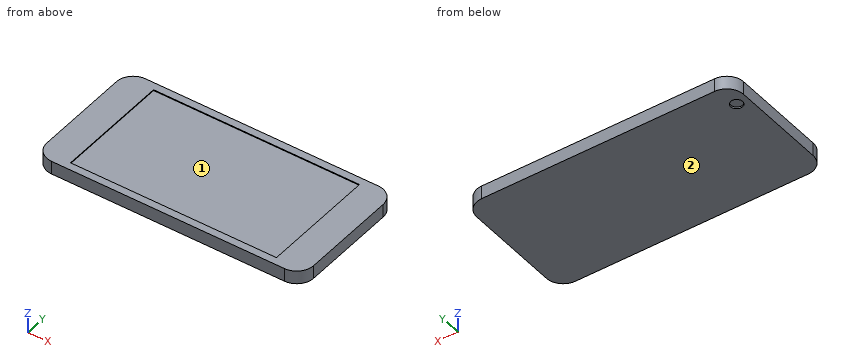
```python
from build123d import *

# Parameters (mm, degrees)
F0_W     = 158
F0_H     = 7.87
F1_DEPTH = 38.435
F2_R     = 10
F3_W     = 122
F3_H     = 68
F4_DEPTH = 0.5
F7_R     = 3.5
F8_DEPTH = 1


# Not quite as in the source:
# - the program builds the solid bodies; features that only make, move or delete a surface that nothing else refers to are left out


with BuildPart() as f1:
    # F0 (on Front) → F1 (new body, symmetric)
    with BuildSketch(Plane.XZ):
        Rectangle(F0_W, F0_H)
    extrude(amount=F1_DEPTH, both=True)

    # F2
    f2_edges = [f1.edges().sort_by_distance(p)[0] for p in [
        (-79, 38.435, 0),
        (-79, -38.435, 0),
        (79, -38.435, 0),
        (79, 38.435, 0),
    ]]
    fillet(f2_edges, radius=F2_R)

    # F3 (on face) → F4 (cut)
    with BuildSketch(Plane.XY.offset(3.935)):
        Rectangle(F3_W, F3_H)
    extrude(amount=-F4_DEPTH, mode=Mode.SUBTRACT)

    # F7 (on face) → F8 (cut)
    with BuildSketch(Plane(origin=(0, 0, -3.935), x_dir=(1, 0, 0), z_dir=(0, 0, -1))):
        with Locations((-72, -24.435)):
            Circle(F7_R)
    extrude(amount=-F8_DEPTH, mode=Mode.SUBTRACT)


solid = f1.part
```
Read the model definition and answer for the solid it produces. Units are mm, in the model's axes. Face numbers are marked on the shaded views. Coordinates: 2 decimals unless noted, no trailing zeros. Loops run counter-clockwise (first coordinate to the right, second up) from the corner with the lowest first, then second, coordinate; pieces in that order, holes last. Notation, with made-up numbers: (70.5, 51.25) -> (74.5, 51.25) arc R5 cw to (74.5, 57.25) -> close; hole circle Ø4 at (61.25, 47.5). An arc over 180 degrees is marked (long way). Return JSON: item names as keys, results as strings.
Item 1: For a pull along X with two mould halves and no side action, classify the marked faces 1 and 2 as +X half, -X half, draft (parallel to the pull), parting line (faces both ways), or undercut.
Answers:
{"face 1": "undercut", "face 2": "draft"}
Item 2: Find section A-A (x = 52.5). Determine the outline of the cut face in (y, z) (3 decimals), plus the area to 3 significant figures.
Answers:
{"outline": "(-38.435, -3.935) -> (38.435, -3.935) -> (38.435, 3.935) -> (34, 3.935) -> (34, 3.435) -> (-34, 3.435) -> (-34, 3.935) -> (-38.435, 3.935) -> close", "area": "571 mm2"}
Item 3: Find the intervals of material crossed by probe 1 along Z at (x, y) = (37, 33.5) (3 decimals); probe 2 along Y at (x, z) = (-72, -3.35) (3 decimals); probe 3 along X at (y, z) = (33, 2.25), in increasing order.
Answers:
{"probe 1": "z = -3.935 to 3.435", "probe 2": "y = -37.974 to 20.935, 27.935 to 37.974", "probe 3": "x = -77.9 to 77.9"}
Item 4: Find section B-B (y = 4.5). Determine the outline of the cut face in (x, z) (3 decimals).
Answers:
{"outline": "(-79, -3.935) -> (79, -3.935) -> (79, 3.935) -> (61, 3.935) -> (61, 3.435) -> (-61, 3.435) -> (-61, 3.935) -> (-79, 3.935) -> close"}
Item 5: Flat-ended cylindrical pins translate along their axes: P1, Ø2, axis at x = -72.5, y = 26, coming from the -Z side (3 decimals); P2, Ø4, axis at x = 22.5, y = 27, coming from the +Z side (3 decimals). Find the tip coordinate at first contact, or state that the pin passes through.
Answers:
{"P1": "stops at z = -2.935", "P2": "stops at z = 3.435"}
Item 6: Find section C-C (y = 23). Determine the outline of the cut face in (x, z) (3 decimals), plus the area to 3 significant figures.
Answers:
{"outline": "(-79, -3.935) -> (-75.192, -3.935) -> (-75.192, -2.935) -> (-68.808, -2.935) -> (-68.808, -3.935) -> (79, -3.935) -> (79, 3.935) -> (61, 3.935) -> (61, 3.435) -> (-61, 3.435) -> (-61, 3.935) -> (-79, 3.935) -> close", "area": "1,180 mm2"}
